```python
from build123d import *

# Parameters (mm, degrees)
SKETCH_1_W          = 6
SKETCH_1_H          = 2
SKETCH_1_H_2        = 10
EXTRUDE_1_DEPTH     = 30
SKETCH_2_W          = 1
SKETCH_2_H          = 17.803492696
CUT_EXTRUDE_1_DEPTH = 30
SKETCH_3_R          = 1.003337712
SKETCH_3_R_2        = 0.930822741
CUT_EXTRUDE_2_DEPTH = 30
FILLET_1_R          = 1


with BuildPart() as part:
    # 草图1 → 凸台-拉伸1 (new body)
    with BuildSketch(Plane.XY):
        with Locations((0, 11)):
            Rectangle(SKETCH_1_W, SKETCH_1_H)
        Polygon((-10, -10), (-10, 10), (-3, 10), (-3, 12), (-12, 12), (-12, -12), (12, -12), (12, 12), (3, 12), (3, 10), (10, 10), (10, -10), align=None)
        with Locations((0, 17)):
            Rectangle(SKETCH_1_W, SKETCH_1_H_2)
    extrude(amount=EXTRUDE_1_DEPTH)

    # 草图2 → 切除-拉伸1 (cut)
    with BuildSketch(Plane.XY.offset(30)):
        with Locations((0, 18.381427763)):
            Rectangle(SKETCH_2_W, SKETCH_2_H)
    extrude(amount=-CUT_EXTRUDE_1_DEPTH, mode=Mode.SUBTRACT)

    # 草图3 → 切除-拉伸2 (cut)
    with BuildSketch(Plane.ZY.offset(3)):
        with Locations(Location((5, 17, 0), (0, 0, 90))):
            Circle(SKETCH_3_R)
        with Locations(Location((25, 17, 0), (0, 0, 90))):
            Circle(SKETCH_3_R_2)
    extrude(amount=-CUT_EXTRUDE_2_DEPTH, mode=Mode.SUBTRACT)

    # 圆角1
    fillet_1_edges = [part.edges().sort_by_distance(p)[0] for p in [
        (12, 0, 0),
        (0, -12, 0),
        (-12, 0, 0),
        (-7.5, 12, 0),
        (-3, 17, 0),
        (3, 17, 0),
        (7.5, 12, 0),
        (12, 12, 15),
        (12, -12, 15),
        (-12, -12, 15),
        (-12, 12, 15),
        (-3, 12, 15),
        (-3, 22, 15),
        (3, 22, 15),
        (3, 12, 15),
        (7.5, 12, 30),
        (3, 17, 30),
        (-3, 17, 30),
        (-7.5, 12, 30),
        (-12, 0, 30),
        (0, -12, 30),
        (12, 0, 30),
    ]]
    fillet(fillet_1_edges, radius=FILLET_1_R)


solid = part.part
```
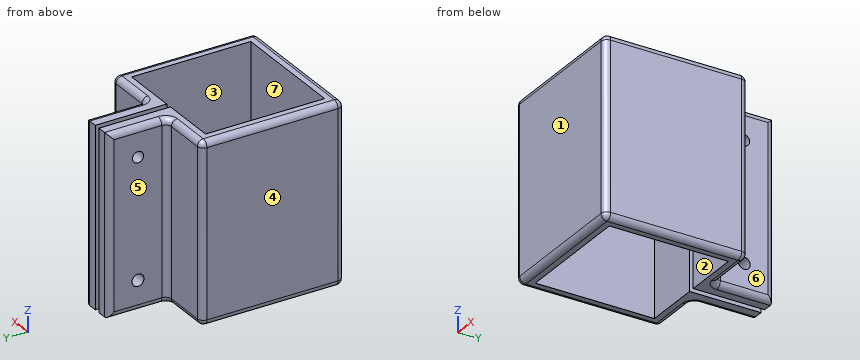
The listing builds one solid part. Answer for the finished solid, in the listing's coordinates (mm). Face numbers are marked on the shaded views. A direction names the side the tool comes from. Round coordinates to 2 decimals unless told otherwise and drop trailing zeros. Write each loop counter-clockwise with the first axis right and the second up, starting at its lowest first coordinate (ties: lowest second). Pieces come first, ordered by that corner, then holes. Notation, with made-up numbers: (-9, 41.25) -> (32, 41.25) arc R32 cw to (32, 77.25) -> close; hole circle Ø7 at (1.5, 4). An arc over 180 degrees is marked (long way). Answer as a JSON object with one key per item and string values. Group by question number.
Q1. Section D-D (y = 10.5) is taken. Write down the section's boundary in (x, z), plus the area to 3 significant figures.
Q2. Section A-A (y = 17) is taken. Write down the section's boundary in (x, z).
Q3. Determine the mould class of the marked faces 1, 2, 3 and 4 for opening direction X: pulls with the +X half, pulls with the -X half, needs draft (parallel to the pull), parting line crosses it, or undercut.
Q4. Each of these flat-tipped pins is pushed along its axis until it touches: pin 1 Ø1.6 at (y, z) = (17, 5) entering from -X; pin 2 Ø2 at (x, z) = (-8, 11.5) entering from +Y; pin 3 Ø6.5 at (y, z) = (16.5, 19.5) entering from -X; pin 4 Ø3 at (y, z) = (17, 25) entering from +X. Where does it stop, or does it pass through?
Q5. Straight lines are drawn through the part: line 1 along Y through (x, z) = (1.8, 25); line 2 along Z through (x, y) = (1.7, 17); line 3 along Y through (x, z) = (7, 26.75). For each, find the intervals that lie inside material, in ascending order.
Q6. Section C-C (x = 7.75) is taken. Write down the section's boundary in (y, z).
Q7. Section B-B (z = 25) is taken. Count the separate pieces of the cut face and the enclosed holes in it, plus the area to 3 significant figures.
Q8. Which of the six approach directions +Z, -Z, +X, -X, +Y, -Y give full straight-line access (tool end or side, diameter ignored) to the marked faces 5, 6 and 7?
Check values:
{
 "1": {"outline": "(-12, 1) arc R1 ccw to (-11, 0) -> (-0.5, 0) -> (-0.5, 30) -> (-11, 30) arc R1 ccw to (-12, 29) -> close; (0.5, 0) -> (11, 0) arc R1 ccw to (12, 1) -> (12, 29) arc R1 ccw to (11, 30) -> (0.5, 30) -> close", "area": "689 mm^2"},
 "2": {"outline": "(-3, 1) arc R1 ccw to (-2, 0) -> (-0.5, 0) -> (-0.5, 4) -> (-3, 4) -> close; (-3, 6) -> (-0.5, 6) -> (-0.5, 24.07) -> (-3, 24.07) -> close; (-3, 25.93) -> (-0.5, 25.93) -> (-0.5, 30) -> (-2, 30) arc R1 ccw to (-3, 29) -> close; (0.5, 0) -> (2, 0) arc R1 ccw to (3, 1) -> (3, 4) -> (0.5, 4) -> close; (0.5, 6) -> (3, 6) -> (3, 24.07) -> (0.5, 24.07) -> close; (0.5, 25.93) -> (3, 25.93) -> (3, 29) arc R1 ccw to (2, 30) -> (0.5, 30) -> close"},
 "3": {"face 1": "needs draft", "face 2": "undercut", "face 3": "undercut", "face 4": "pulls with the -X half"},
 "4": {"pin 1": "through", "pin 2": "y = 12", "pin 3": "x = -3", "pin 4": "x = 3"},
 "5": {"line 1": "-12 to -10, 10 to 16.07, 17.93 to 22", "line 2": "0 to 4, 6 to 24.07, 25.93 to 30", "line 3": "-12 to -10, 10 to 12"},
 "6": {"outline": "(-12, 1) arc R1 ccw to (-11, 0) -> (-10, 0) -> (-10, 30) -> (-11, 30) arc R1 ccw to (-12, 29) -> close; (10, 0) -> (11, 0) arc R1 ccw to (12, 1) -> (12, 29) arc R1 ccw to (11, 30) -> (10, 30) -> close"},
 "7": {"separate pieces": "3", "enclosed holes": "0", "area": "214 mm^2"},
 "8": {"face 5": "+Z, -Z, -X, +Y", "face 6": "+Z, -Z, +X, +Y", "face 7": "+Z, -Z"}
}
